Verification items for the finished model (mm, model axes). A direction names the side the tool comes from. Give positions to 0.01 mm unless a question says otherwise; leave off trailing zeros. Write each loop counter-clockwise with the first axis right and the second up, starting at its lowest first coordinate (ties: lowest second). Pieces come first, ordered by that corner, then holes.
Autodesk Inventor part; units mm, degrees
ref_plane "Work Plane1" through (-48.2558, -133.096, 27.8605) normal (-0.5, 0, -0.866) x (-0.866, 0, 0.5)
ref_plane "Work Plane3" through (-43.4442, -113.7031, -25.0825) normal (0.866, 0, 0.5) x (0, 1, 0)
ref_plane "YZ Plane" through (0, 0, 0) normal (1, 0, 0) x (0, 1, 0)
sketch "Sketch1" plane through (0, 0, 0) normal (0, 1, 0) x (-1, 0, 0)
  circle A0 centre (0, 0) radius 50.8
  dimension "d0" = 101.6
extrude "Extrusion1" add sketch "Sketch1" along normal blind 7.62
sketch "Sketch2" plane through (0, 7.62, 0) normal (0, 1, 0) x (1, 0, 0)
  circle A0 centre (0, 0) radius 49.2125
  circle A1 centre (0, 0) radius 50.8
  dimension "d3" = 98.425
extrude "Extrusion2" cut sketch "Sketch2" against normal blind 3.175
sketch "Sketch3" plane through (0, 7.62, 0) normal (0, 1, 0) x (1, 0, 0)
  circle A0 centre (0, 0) radius 50.9584
extrude "Extrusion3" add sketch "Sketch3" along normal blind 7.62
sketch "Sketch4" plane through (0, 15.24, 0) normal (0, 1, 0) x (1, 0, 0)
  point P0 (0, 0)
sketch "Sketch5" plane through (0, 15.24, 0) normal (0, 1, 0) x (1, 0, 0)
  circle A0 centre (0, 0) radius 49.2125
  circle A1 centre (0, 0) radius 50.9584
  dimension "d8" = 98.425
extrude "Extrusion4" cut sketch "Sketch5" against normal blind 3.175
sketch "Sketch6" plane through (0, 15.24, 0) normal (0, 1, 0) x (1, 0, 0)
  circle A0 centre (0, 0) radius 50.8
  dimension "d11" = 101.6
extrude "Extrusion5" add sketch "Sketch6" along normal blind 5.08
sketch "Sketch7" plane through (0, 0, 0) normal (0, -1, 0) x (1, 0, 0)
  circle A0 centre (0, 0) radius 57.15
  dimension "d14" = 114.3
extrude "Extrusion6" add sketch "Sketch7" along normal blind 6.096
chamfer "Chamfer1" distance 2.54 angle 45 1 edges at (-50.8, 20.32, 0)
sketch "Sketch8" plane through (0, -6.096, 0) normal (0, -1, 0) x (1, 0, 0)
  circle A0 centre (0, 0) radius 50.8
  circle A1 centre (53.975, 0) radius 1.7526
  circle A2 centre (26.9875, 46.7437) radius 1.7526
  circle A3 centre (-26.9875, 46.7437) radius 1.7526
  circle A4 centre (-53.975, 0) radius 1.7526
  circle A5 centre (-26.9875, -46.7437) radius 1.7526
  circle A6 centre (26.9875, -46.7437) radius 1.7526
  dimension "d20" = 3.5052
  dimension "d21" = 53.975
  dimension "d24" = 360
extrude "Extrusion7" cut sketch "Sketch8" against normal blind 6.096 contours A1 | A2 | A3 | A4 | A5 | A6
sketch "Sketch9" plane through (0, -6.096, 0) normal (0, -1, 0) x (1, 0, 0)
  circle A0 centre (0, 0) radius 12.7
  circle A1 centre (0, 0) radius 1.27
  dimension "d28" = 25.4
  dimension "d29" = 2.54
extrude "Extrusion8" cut sketch "Sketch9" against normal blind 127 contours A1
sketch "Sketch10" plane through (0, -6.096, 0) normal (0, -1, 0) x (1, 0, 0)
  circle A0 centre (0, 0) radius 1.27
  circle A1 centre (0, 0) radius 38.1
  dimension "d33" = 76.2
extrude "Extrusion9" cut sketch "Sketch10" against normal blind 9.525
sketch "Sketch11" plane through (0, 3.429, 0) normal (0, -1, 0) x (1, 0, 0)
  circle A0 centre (0, 0) radius 12.7
  circle A1 centre (0, 0) radius 1.27
  dimension "d36" = 25.4
extrude "Extrusion10" add sketch "Sketch11" along normal blind 9.525
sketch "Sketch12" plane through (0, 20.32, 0) normal (0, 1, 0) x (1, 0, 0)
  circle A0 centre (0, 0) radius 1.27
  circle A1 centre (0, 0) radius 38.1
extrude "Extrusion11" cut sketch "Sketch12" against normal blind 508
sketch "Sketch13" plane through (0, -6.096, 0) normal (0, -1, 0) x (1, 0, 0)
  point P0 (0, 0)
sketch "Sketch14" plane through (0, -6.096, 0) normal (0, -1, 0) x (1, 0, 0)
  line L0 (0, -60.96) -> (12.7, -60.96)
  line L1 (0, -60.96) -> (-12.7, -60.96)
  circle A0 centre (0, 0) radius 57.15
  arc A1 (-12.7, -55.721) -> (12.7, -55.721) centre (0, 0) ccw
  line L2 (12.7, -60.96) -> (12.7, -55.721)
  line L3 (-12.7, -60.96) -> (-12.7, -55.721)
  line L4 (52.7929, 30.48) -> (59.1429, 19.4815)
  line L5 (52.7929, 30.48) -> (46.4429, 41.4785)
  line L6 (46.4429, 41.4785) -> (41.9058, 38.859)
  arc A2 (54.6058, 16.862) -> (41.9058, 38.859) centre (0, 0) ccw
  line L7 (59.1429, 19.4815) -> (54.6058, 16.862)
  line L8 (-52.7929, 30.48) -> (-46.4429, 41.4785)
  line L9 (-52.7929, 30.48) -> (-59.1429, 19.4815)
  line L10 (-59.1429, 19.4815) -> (-54.6058, 16.862)
  arc A3 (-41.9058, 38.859) -> (-54.6058, 16.862) centre (0, 0) ccw
  line L11 (-46.4429, 41.4785) -> (-41.9058, 38.859)
  point P0 (0, -57.15)
  point P1 (49.4934, 28.575)
  point P2 (-49.4934, 28.575)
  dimension "d41" = 12.7
  dimension "d42" = 12.7
  dimension "d43" = 3.81
  dimension "d46" = 360
extrude "Extrusion12" add sketch "Sketch14" along normal blind 127 and the other way blind 5.08 contours L1 L3 A0 L2 L0 | L10 L9 L8 L11 A0 | A0 L6 L5 L4 L7
chamfer "Chamfer2" distance 3.175 angle 45 3 edges at (52.7929, -1.016, 30.48) (0, -1.016, -60.96) (-52.7929, -1.016, 30.48)
fillet "Fillet1" radius 3.175 6 edges at (-59.1429, -68.6435, 19.4815) (-46.4429, -68.6435, 41.4785) (-12.7, -68.6435, -60.96) (12.7, -68.6435, -60.96) (59.1429, -68.6435, 19.4815) (46.4429, -68.6435, 41.4785)
ref_plane "Work Plane1" through (-48.2558, -133.096, 27.8605) normal (-0.5, 0, -0.866) x (-0.866, 0, 0.5)
sketch "Sketch15" plane through (-48.2558, -133.096, 27.8605) normal (-0.5, 0, -0.866) x (-0.866, 0, 0.5)
  line L0 (-55.721, 148.3202) -> (-55.721, -8.2891)
  line L1 (1.429, 0) -> (0, 0)
  line L2 (1.429, 0) -> (-1.111, 0)
  line L3 (-1.111, 0) -> (-1.111, 38.7858)
  line L4 (-1.111, 38.7858) -> (1.429, 38.7858)
  line L5 (1.429, 38.7858) -> (1.429, 0)
  point P0 (-55.721, 133.096)
  dimension "d58" = 2.54
  dimension "d59" = 38.7858
revolve "Revolution1" add sketch "Sketch15" angle 360 about axis through (0, 15.2242, 0) along (0, -1, 0)
ref_plane "Work Plane3" through (-43.4442, -113.7031, -25.0825) normal (0.866, 0, 0.5) x (0, 1, 0)
ref_plane "Work Plane2" through (47.2936, -113.7031, 27.305) normal (0.866, 0, 0.5) x (0, 1, 0)
sketch "Sketch16" plane through (-43.4442, -113.7031, -25.0825) normal (0.866, 0, 0.5) x (0, 1, 0)
  line L0 (19.3929, 41.9058) -> (19.3929, -41.9058)
  line L1 (19.3929, 0) -> (-60.7336, 0)
  line L2 (19.3929, 54.6058) -> (-19.3929, 54.6058)
  line L3 (0, 54.6058) -> (0, -48.0304)
  line L4 (109.5121, -48.0304) -> (-19.3929, -48.0304)
  circle A0 centre (9.398, 0) radius 1.4986
  circle A1 centre (-9.398, 0) radius 1.4986
  circle A2 centre (0, -9.398) radius 1.4986
  circle A3 centre (0, 9.398) radius 1.4986
  point P0 (113.7031, 0)
  dimension "d64" = 2.9972
  dimension "d65" = 2.9972
  dimension "d66" = 2.9972
  dimension "d67" = 2.9972
  dimension "d68" = 18.796
  dimension "d69" = 18.796
  dimension "d70" = 18.796
  dimension "d71" = 18.796
extrude "Extrusion13" cut sketch "Sketch16" against normal blind 127
sketch "Sketch17" plane through (0, 20.32, 0) normal (0, 1, 0) x (1, 0, 0)
  circle A0 centre (0, 0) radius 38.1
  circle A1 centre (0, 0) radius 31.75
  circle A2 centre (0, 0) radius 50.8
  dimension "d74" = 6.35
  dimension "d75" = 12.7
extrude "Extrusion14" add sketch "Sketch17" against normal blind 26.416 contours A0
sketch "Sketch18" plane through (48.0304, -133.096, 38.7289) normal (0.866, 0, 0.5) x (0.5, 0, -0.866)
  line L0 (0, 128.905) -> (19.05, 128.905)
  circle A0 centre (9.525, 128.905) radius 1.5
  point P0 (9.525, 133.096)
  dimension "d78" = 3
extrude "Extrusion15" cut sketch "Sketch18" against normal blind 10.16
sketch "Sketch19" plane through (9.525, -133.096, -60.96) normal (0, 0, -1) x (-1, 0, 0)
  line L0 (0, 128.905) -> (19.05, 128.905)
  circle A0 centre (9.525, 128.905) radius 1.5
  point P0 (9.525, 133.096)
  dimension "d81" = 3
extrude "Extrusion16" cut sketch "Sketch19" against normal blind 10.16
sketch "Sketch20" plane through (-48.0304, -133.096, 38.7289) normal (-0.866, 0, 0.5) x (0.5, 0, 0.866)
  line L0 (-19.05, 128.905) -> (0, 128.905)
  circle A0 centre (-9.525, 128.905) radius 1.5
  point P0 (-9.525, 133.096)
  dimension "d84" = 3
extrude "Extrusion17" cut sketch "Sketch20" against normal blind 10.16
sketch "Sketch21" plane through (0, -6.096, 0) normal (0, -1, 0) x (1, 0, 0)
  circle A0 centre (0, 0) radius 57.15
  circle A1 centre (0, 0) radius 50.8
  circle A2 centre (0, 0) radius 64.3517
extrude "Extrusion18" cut sketch "Sketch21" along normal blind 304.8 and the other way blind 304.8 contours A2
sketch "Sketch22" plane through (0, -133.096, 0) normal (0, -1, 0) x (1, 0, 0)
  circle A0 centre (0, 0) radius 54.61
  circle A1 centre (0, 0) radius 57.15
extrude "Extrusion19" cut sketch "Sketch22" against normal blind 50.8
sketch "Sketch23" plane through (0, 20.32, 0) normal (0, 1, 0) x (1, 0, 0)
  circle A0 centre (0, 0) radius 31.75
  circle A1 centre (0, 0) radius 48.26
  circle A2 centre (-36.83, -15.6083) radius 1.5
  circle A3 centre (-36.83, 15.6083) radius 1.5
  circle A4 centre (36.83, -15.6083) radius 1.5
  circle A5 centre (36.83, 15.6083) radius 1.5
  line L0 (-36.83, -14.1083) -> (-36.83, 14.1083)
  line L1 (36.83, -14.1083) -> (36.83, 14.1083)
  point P0 (-36.83, 0)
  point P1 (36.83, 0)
  point P2 (-36.83, 0)
  point P3 (36.83, 0)
  dimension "d93" = 3
  dimension "d95" = 3
  dimension "d96" = 3
  dimension "d97" = 3
  dimension "d94" = 73.66
  dimension "d98" = 31.2166
  dimension "d99" = 31.2166
extrude "Extrusion20" cut sketch "Sketch23" against normal blind 10.16 contours A2 | A3 | A4 | A5
sketch "Sketch24" plane through (0, 20.32, 0) normal (0, 1, 0) x (1, 0, 0)
  circle A0 centre (36.83, 15.6083) radius 1.5
  circle A1 centre (36.83, 15.6083) radius 1.5
  circle A2 centre (36.83, -15.6083) radius 1.5
  circle A3 centre (36.83, -15.6083) radius 1.5
  circle A4 centre (-36.83, -15.6083) radius 1.5
  circle A5 centre (-36.83, -15.6083) radius 1.5
  circle A6 centre (-36.83, 15.6083) radius 1.5
  circle A7 centre (-36.83, 15.6083) radius 1.5
  line L0 (0, 0) -> (36.83, 0)
  line L1 (36.83, 0) -> (36.83, 15.6083)
  dimension "d102" = 36.83
  dimension "d103" = 15.6083
equation "\"d42\" = d41"
equation "\"d65\" = d64"
equation "\"d66\" = d65"
equation "\"d67\" = d64"
equation "\"d68\" = d69"
equation "\"d71\" = d70"
equation "\"d95\" = d93"
equation "\"d96\" = d93"
equation "\"d97\" = d96"
properties part number "O ring fitting connecting with the Control Board"
Item 1: Set-up check for faces 4 (the face through (-26.045, -3.091, -45.266)), 5 (the face through (0, -4, -50.8)), 6 (the face through (37, 10.16, -16)), 7 (the face through (11.012, 2.191, 49.592)): record each of +Z, -Z, +X, -X, +Y, -Y from which the full face is reachable in a straight line by a thin tool's end or side.
Answer key:
face 4: +Y, -Y
face 5: -Z
face 6: +Y
face 7: none
Item 2: Sectioned sample at C-C on z = 0. State how many separate pieces and enclosed holes the cut face has, then the cut area to 3 significant figures.
Answer key:
separate pieces: 4
enclosed holes: 0
area: 1,020 mm2
Item 3: Scan lines: line 1 along Z through (x, y) = (0.5, -2.5); line 2 along Y through (x, z) = (-40.5, 35.5); line 3 along Z through (x, y) = (-17, 3). Record each from-to range of solid material in increasing order.
Answer key:
line 1: z = -57.15 to -31.75, 31.75 to 57.15
line 2: y = -6.1 to 0
line 3: z = -47.87 to -26.82, 26.82 to 47.87
Item 4: Sectioned sample at B-B on y = 2. Record the cut outline in (x, z), then the cut area to 3 significant figures.
Answer key:
outline: circle Ø101.6 at (0, 0); hole circle Ø63.5 at (0, 0)
area: 4,940 mm2
Item 5: Release check for a two-part mould opening along X. For faces 1 (the face through (-11.012, 16.492, -49.592)), 2 (the face through (-36.024, 15.311, 14.343)), 3 (the face through (25, -6.096, 25)) record: released by +X, released by -X, zero draft, split by the parting line, or undercut.
Answer key:
face 1: split by the parting line
face 2: undercut
face 3: zero draft
Item 6: Depth check by flat-ended pin: pin 1 (4 mm diameter, centred on y = 17, z = 34, fed in from -X); pin 2 (1.5 mm diameter, centred on x = 37, z = 15.5, fed in from +Y); pin 3 (3 mm diameter, centred on x = -53.975, z = 0, fed in from +Y); pin 4 (8 mm diameter, centred on y = 3, z = -44, fed in from +X). Enter the tip coordinate at first touch or a pass-through.
Answer key:
pin 1: stops at x = -39.45
pin 2: stops at y = 10.16
pin 3: passes through
pin 4: stops at x = 39.45
